Solid Edge part; units mm, degrees
sketch "Sketch1" plane through (0, 0, 0) normal (0, 0, 1) x (1, 0, 0)
  line L0 (0.623, 12.25) -> (0.8305, 12.25)
  line L1 (0.8305, 12.25) -> (1.038, 14.875)
  line L2 (1.038, 14.875) -> (1.038, 16.1629)
  line L3 (1.038, 16.1629) -> (0.8305, 17.5)
  line L4 (0.8305, 17.5) -> (0.623, 17.5)
  line L5 (0.623, 17.5) -> (0.7268, 16.1875)
  line L6 (0.7268, 16.1875) -> (0.623, 14.875)
  line L7 (0.623, 14.875) -> (0.623, 12.25)
revolve "RevolvedProtrusion1" add sketch "Sketch1" angle 360 about axis through (0.8305, 0, 0) along (-1, 0, 0)
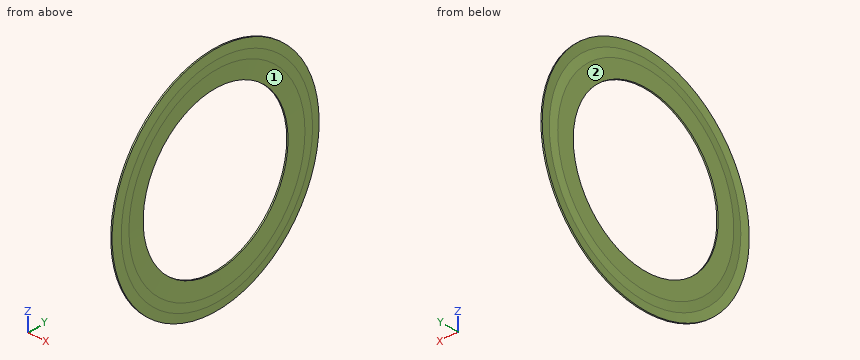
Geometry: final body of the model. Coordinates: model frame, mm. Face numbers are marked on the shaded views. Coordinates: 2 decimals unless noted, no trailing zeros. Order: outer loops, then holes, each group sorted by start corner. A loop starts at its lowest first (then second) coordinate and runs counter-clockwise, first axis right, second up. Notation, with made-up numbers: (6.5, 50.5) - (46.5, 50.5) arc R22 ccw to (46.5, 69.5) - close; hole circle Ø9 at (72.5, 34.5). An arc over 180 degrees is marked (long way). Return JSON: item names as keys, results as strings. Group by question number.
1. Pull-direction query (Z, two-part tool) for the marked faces 1 and 2; classes: pulls with the +Z half, pulls with the -Z half, needs draft (parallel to the pull), parting line crosses it, or undercut.
2. Material intervals for line 1 along Y through (x, z) = (0.8, -2); line 2 along Z through (x, y) = (0.8, -10), sorted ascending. Write a range as [from, to].
3. Cut plane C-C (x = 0.9). Output: boundary loops of the cut face in (y, z), plus the area to 3 significant figures.
Resolved:
{
 "1": {"face 1": "undercut", "face 2": "needs draft"},
 "2": {"line 1": "y = [-17.39, -12.09], [12.09, 17.39]", "line 2": "z = [-14.36, -7.08], [7.08, 14.36]"},
 "3": {"outline": "circle Ø34.1 at (0, 0); hole circle Ø26.26 at (0, 0)", "area": "372 mm²"}
}
